Can you work these out from the model? Positions are in its coordinate system, mm. Face numbers are marked on the shaded views. A direction names the side the tool comes from. Coordinates: 2 decimals unless noted, no trailing zeros. Order: outer loops, then holes, each group sorted by start corner. A loop starts at its lowest first (then second) coordinate and runs counter-clockwise, first axis right, second up. Notation, with made-up numbers: (-25.5, 66.25) -> (10.5, 66.25) arc R36 ccw to (10.5, 101.25) -> close; hole circle Ø8 at (-1.75, -12). An arc over 180 degrees is marked (long way). Use a Markdown table: item, result. Add a question column.
1. Suppose I cut it at B-B, the plane x = 5.5. List the corners of the cut face in (y, z) for me.
2. For pin 1 Ø6 at (x, z) = (16.5, 14) entering from +Y; pin 2 Ø10 at (y, z) = (13, 18.5) entering from +X, each with a flat end and sliding along its axis, tell me the tip position at first contact or that it passes through.
3. Suppose I cut it at D-D, the plane z = 30. List the corners of the cut face in (x, y) for me, then the cut area to 3 significant figures.
4. For the marked faces 1 and 2, which set-ups out of +Z, -Z, +X, -X, +Y, -Y let a thin tool reach every point of the face, with its end or its side?
5. Suppose I cut it at C-C, the plane y = 16. List the corners of the cut face in (x, z) for me.
6. Suppose I cut it at A-A, the plane z = 10. List the corners of the cut face in (x, y) for me, then the cut area to 3 significant figures.
7. If I drill on line 1 along Y through (x, z) = (0.6, 10); line 2 along X through (y, z) = (16.5, 15), over which ranges is the centre line in solid material (lowest first)? Write a range as from..to.
```python
from build123d import *

# Parameters (mm, degrees)
BOSS_EXTRUDE1_DEPTH = 40
SKETCH2_W           = 28
SKETCH2_H           = 3
CUT_EXTRUDE1_DEPTH  = 10
SKETCH3_R           = 1.5
CUT_EXTRUDE2_DEPTH  = 10


with BuildPart() as part:
    # Sketch1 → Boss-Extrude1 (new body)
    with BuildSketch(Plane.XY):
        Polygon((0, 0), (35, 0), (35, 1), (1, 1), (1, 20), (0, 20), align=None)
    extrude(amount=BOSS_EXTRUDE1_DEPTH)

    # Sketch2 → Cut-Extrude1 (cut)
    with BuildSketch(Plane(origin=(0, 1, 0), x_dir=(1, 0, 0), z_dir=(0, 1, 0))):
        with Locations((16, -8)):
            Rectangle(SKETCH2_W, SKETCH2_H)
        with Locations((16, -31)):
            Rectangle(SKETCH2_W, SKETCH2_H)
    extrude(amount=-CUT_EXTRUDE1_DEPTH, mode=Mode.SUBTRACT)

    # Sketch3 → Cut-Extrude2 (cut)
    with BuildSketch(Plane.ZY):
        with Locations((30, 16)):
            Circle(SKETCH3_R)
        with Locations((10, 16)):
            Circle(SKETCH3_R)
    extrude(amount=-CUT_EXTRUDE2_DEPTH, mode=Mode.SUBTRACT)


solid = part.part
```
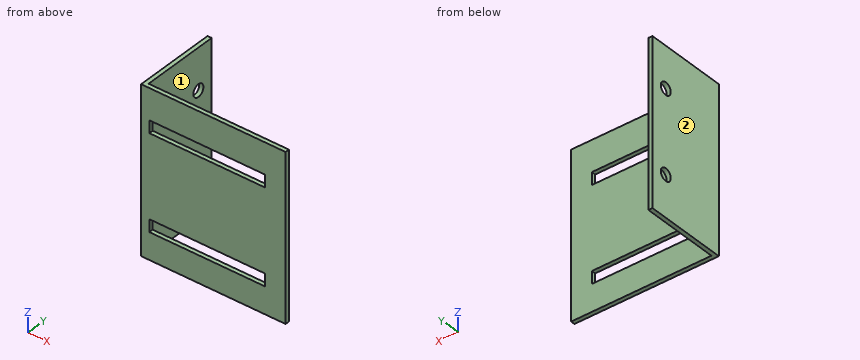
Worked out:
| question | item | result |
|---|---|---|
| 1 | outline | (0, 0) -> (1, 0) -> (1, 6.5) -> (0, 6.5) -> close; (0, 9.5) -> (1, 9.5) -> (1, 29.5) -> (0, 29.5) -> close; (0, 32.5) -> (1, 32.5) -> (1, 40) -> (0, 40) -> close |
| 2 | pin 1 | stops at y = 1 |
| 2 | pin 2 | stops at x = 1 |
| 3 | outline | (0, 0) -> (2, 0) -> (2, 1) -> (1, 1) -> (1, 14.5) -> (0, 14.5) -> close; (0, 17.5) -> (1, 17.5) -> (1, 20) -> (0, 20) -> close; (30, 0) -> (35, 0) -> (35, 1) -> (30, 1) -> close |
| 3 | area | 23.0 mm² |
| 4 | face 1 | +Z, -Z, +X, +Y |
| 4 | face 2 | +Z, -Z, -X, +Y, -Y |
| 5 | outline | (0, 0) -> (1, 0) -> (1, 8.5) -> (0, 8.5) -> close; (0, 11.5) -> (1, 11.5) -> (1, 28.5) -> (0, 28.5) -> close; (0, 31.5) -> (1, 31.5) -> (1, 40) -> (0, 40) -> close |
| 6 | outline | (0, 0) -> (35, 0) -> (35, 1) -> (1, 1) -> (1, 14.5) -> (0, 14.5) -> close; (0, 17.5) -> (1, 17.5) -> (1, 20) -> (0, 20) -> close |
| 6 | area | 51.0 mm² |
| 7 | line 1 | y = 0..14.5, 17.5..20 |
| 7 | line 2 | x = 0..1 |
